Read the model definition and answer for the solid it produces. Units are mm, in the model's axes. A direction names the side the tool comes from. Round coordinates to 2 decimals unless told otherwise and drop trailing zeros. Order: outer loops, then holes, each group sorted by start corner. A loop starts at its lowest first (then second) coordinate and runs counter-clockwise, first axis right, second up. Notation, with made-up numbers: (-8, 12.5) -> (5, 12.5) arc R13 ccw to (5, 30.5) -> close; hole circle Ø9 at (36, 48). An arc over 180 degrees is marked (long way). Use a Markdown table: item, result. Add a question column.
1. Section C-C, the plane x = 20 is taken. Give the vertices of the cut face in (y, z), then the cut area to 3 significant figures.
2. The mould has two halves that part along X. Classify faces 4 (the face through (27.61, -0.99, -3.51)), 5 (the face through (8.72, -0.99, -11.91)), 6 (the face through (-6.73, -0.99, -14.76)), 7 (the face through (5, 0, -1)): +X half, -X half, draft (parallel to the pull), parting line (faces both ways), or undercut.
3. Section A-A, the plane y = -1.7 is taken. Give the vertices of the cut face in (x, z).
4. Section B-B, the plane z = 0.5 is taken. Give the vertices of the cut face in (x, y).
5. Consider L1, parallel to Z at x = 26, y = -0.8; L2, parallel to Z at x = 27.5, y = -0.1; L3, parallel to X at y = -0.35, z = -8.75. Determine where each line is inside the solid, lowest interval first. Write a range as [from, to].
6. For faces 1 (the face through (11.1, -1, -7.4)), 2 (the face through (26.75, -0.99, 0.22)), 3 (the face through (23.205, -0.986, -3.238)), determine the directions among +Z, -Z, +X, -X, +Y, -Y from which every point of the face is accessible in a straight line to the end or side of a thin tool.
```python
from build123d import *

# Parameters (mm, degrees)
F1_DEPTH = 2
F2_R     = 4
F3_R     = 2


with BuildPart() as f1:
    # F0 (on Front) → F1 (new body)
    with BuildSketch(Plane.XZ):
        Polygon((-10.456731, 12.310552), (-10.456731, -15.486014), (-2.603713, -13.959542), (7.341506, -15.004827), (10.839441, -7.148336), (21.240145, -3.567086), (25.226323, -2.90037), (30.069817, -4.141563), (30.318056, -3.172864), (25.673877, -1.982748), (27.85655, 2.492394), align=None)
    extrude(amount=F1_DEPTH)

    # F2
    f2_edges = [f1.edges().sort_by_distance(p)[0] for p in [
        (10.839441, -1, -7.148336),
    ]]
    fillet(f2_edges, radius=F2_R)

    # F3
    f3_edges = [f1.edges().sort_by_distance(p)[0] for p in [
        (-2.603713, -1, -13.959542),
    ]]
    fillet(f3_edges, radius=F3_R)


solid = f1.part
```
Verdict:
| question | item | result |
|---|---|---|
| 1 | outline | (-2, -3.99) -> (0, -3.99) -> (0, 4.51) -> (-2, 4.51) -> close |
| 1 | area | 17.0 mm2 |
| 2 | face 4 | undercut |
| 2 | face 5 | +X half |
| 2 | face 6 | undercut |
| 2 | face 7 | draft |
| 3 | outline | (-10.46, -15.49) -> (-2.9, -14.02) arc R2 cw to (-2.31, -13.99) -> (7.34, -15) -> (10.13, -8.74) arc R4 cw to (12.48, -6.58) -> (21.24, -3.57) -> (25.23, -2.9) -> (30.07, -4.14) -> (30.32, -3.17) -> (25.67, -1.98) -> (27.86, 2.49) -> (-10.46, 12.31) -> close |
| 4 | outline | (-10.46, -2) -> (26.88, -2) -> (26.88, 0) -> (-10.46, 0) -> close |
| 5 | L1 | z = [-3.1, -2.07], [-1.31, 2.97] |
| 5 | L2 | z = [-3.48, -2.45], [1.76, 2.58] |
| 5 | L3 | x = [-10.46, 10.13] |
| 6 | face 1 | -Z, +X, +Y, -Y |
| 6 | face 2 | +X, +Y, -Y |
| 6 | face 3 | -Z, +Y, -Y |
